Here's how the part is built. I have some questions about the finished solid (model axes, mm). Coordinates: 2 decimals unless noted, no trailing zeros. Write each loop counter-clockwise with the first axis right and the second up, starting at its lowest first coordinate (ties: lowest second). Pieces come first, ordered by that corner, then holes. Notation, with made-up numbers: (-26, 81) - (19, 81) arc R27 ccw to (19, 109) - close; hole circle Ø3 at (85, 19.25). An arc over 180 degrees is marked (long way). Answer in a Markdown table with one row per item. Add a question column.
Item 1: Imagine slicing it at D-D (x = 48). Please give me the cut outline in (y, z), plus the area to 3 significant figures.
Item 2: If I drill on probe 1 along X at (y, z) = (3.15, 0); probe 2 along Z at (x, y) = (11.5, 3.45); probe 3 along X at (y, z) = (3.7, -33.5), over which ranges is the centre line in solid material (lowest first)? Write a range as from..to.
Item 3: Imagine slicing it at B-B (z = 0). Please give me the cut outline in (x, y).
Item 4: Imagine slicing it at C-C (y = 1.25). Please give me the cut outline in (x, z).
Item 5: Imagine slicing it at A-A (x = 0). Please give me the cut outline in (y, z), plus the area to 3 significant figures.
Item 6: I'm going to push flat-ended pins straight in: pin 1 (1.5 mm diameter, centred on x = -31, z = -2.5, fed in from +Y); pin 2 (1 mm diameter, centred on y = 2.5, z = -9, fed in from +X); pin 3 (2 mm diameter, centred on x = 29.5, y = 3.5, fed in from -Z). Where does each tip first touch, or does it pass through?
from build123d import *

# Parameters (mm, degrees)
SKETCH1_R             = 72.5
BOSS_EXTRUDE1_DEPTH   = 6
SKETCH2_R             = 17.5
CUT_EXTRUDE1_DEPTH    = 103.705890776
SKETCH3_R             = 5.721006682
CUT_EXTRUDE2_DEPTH    = 3.69464
CIRPATTERN1_START     = 2.305359648
CIRPATTERN1_OUTLINE_R = 5.721006682
CIRPATTERN1_DEPTH     = 3.694640352


# Read off the part's stored shape, not the designer's step: CirPattern1
with BuildPart() as part:
    # Sketch1 → Boss-Extrude1 (new body)
    with BuildSketch(Plane(origin=(0, 0, 0), x_dir=(1, 0, 0), z_dir=(0, 1, 0))):
        with Locations(Location((0, 0, 0), (0, 0, 270))):
            Circle(SKETCH1_R)
    extrude(amount=BOSS_EXTRUDE1_DEPTH)

    # Sketch2 → Cut-Extrude1 (cut, through all)
    with BuildSketch(Plane(origin=(0, 0, 0), x_dir=(1, 0, 0), z_dir=(0, 1, 0))):
        with Locations(Location((0, 0, 0), (0, 0, 270))):
            Circle(SKETCH2_R)
    extrude(amount=CUT_EXTRUDE1_DEPTH, mode=Mode.SUBTRACT)

    # Sketch3 → Cut-Extrude2 (cut)
    with BuildSketch(Plane(origin=(0, 6, 0), x_dir=(1, 0, 0), z_dir=(0, 1, 0))):
        with Locations(Location((-32.5149274, 0, 0), (0, 0, 270))):
            Circle(SKETCH3_R)
    extrude(amount=-CUT_EXTRUDE2_DEPTH, mode=Mode.SUBTRACT)

    # CirPattern1 outline → CirPattern1 (cut)
    with BuildSketch(Plane(origin=(0, 0, 0), x_dir=(1, 0, 0), z_dir=(0, 1, 0)).offset(CIRPATTERN1_START)):
        with Locations((0, 32.5149274)):
            Circle(CIRPATTERN1_OUTLINE_R)
        with Locations((32.5149274, 0)):
            Circle(CIRPATTERN1_OUTLINE_R)
        with Locations((0, -32.5149274)):
            Circle(CIRPATTERN1_OUTLINE_R)
    extrude(amount=CIRPATTERN1_DEPTH, mode=Mode.SUBTRACT)


solid = part.part
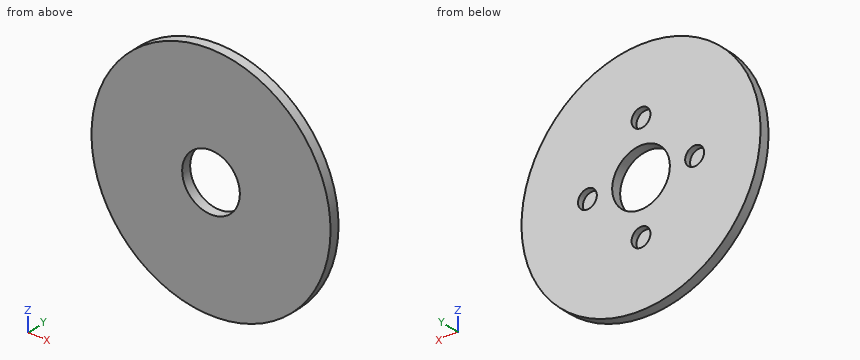
Here are the results:
| question | item | result |
|---|---|---|
| 1 | outline | (0, -54.33) - (6, -54.33) - (6, 54.33) - (0, 54.33) - close |
| 1 | area | 652 mm2 |
| 2 | probe 1 | x = -72.5..-38.24, -26.79..-17.5, 17.5..26.79, 38.24..72.5 |
| 2 | probe 2 | z = -71.58..-13.19, 13.19..71.58 |
| 2 | probe 3 | x = -64.3..-5.64, 5.64..64.3 |
| 3 | outline | (-72.5, 0) - (-17.5, 0) - (-17.5, 6) - (-26.79, 6) - (-26.79, 2.31) - (-38.24, 2.31) - (-38.24, 6) - (-72.5, 6) - close; (17.5, 0) - (72.5, 0) - (72.5, 6) - (38.24, 6) - (38.24, 2.31) - (26.79, 2.31) - (26.79, 6) - (17.5, 6) - close |
| 4 | outline | circle Ø145 at (0, 0); hole circle Ø35 at (0, 0) |
| 5 | outline | (0, -72.5) - (6, -72.5) - (6, -38.24) - (2.31, -38.24) - (2.31, -26.79) - (6, -26.79) - (6, -17.5) - (0, -17.5) - close; (0, 17.5) - (6, 17.5) - (6, 26.79) - (2.31, 26.79) - (2.31, 38.24) - (6, 38.24) - (6, 72.5) - (0, 72.5) - close |
| 5 | area | 575 mm2 |
| 6 | pin 1 | stops at y = 2.31 |
| 6 | pin 2 | stops at x = 72 |
| 6 | pin 3 | stops at z = -66.66 |
